from build123d import *

# Parameters (mm, degrees)
SKETCH1_R           = 2.25
BOSS_EXTRUDE1_DEPTH = 25
BOSS_EXTRUDE2_DEPTH = 4
CHAMFER1_SIZE       = 0.5


with BuildPart() as part:
    # Sketch1 → Boss-Extrude1 (new body)
    with BuildSketch(Plane.XY):
        Circle(SKETCH1_R)
    extrude(amount=BOSS_EXTRUDE1_DEPTH)

    # Sketch2 → Boss-Extrude2 (add)
    with BuildSketch(Plane.XY.offset(25)):
        Polygon((1.886184201, 3.57767771), (-2.155267683, 3.42232229), (-4.041451884, -0.15535542), (-1.886184201, -3.57767771), (2.155267683, -3.42232229), (4.041451884, 0.15535542), align=None)
    extrude(amount=BOSS_EXTRUDE2_DEPTH)

    # Sketch4 → Cut-Revolve1 (revolve, cut)
    with BuildSketch(Plane(origin=(0, 0, 0), x_dir=(1, 0, 0), z_dir=(0, 1, 0))):
        with BuildLine():
            Line((4.041451884, -28.3), (4.041451884, -29))
            Line((4.041451884, -29), (3.341451884, -29))
            ThreePointArc((3.341451884, -29), (3.836426631, -28.794974747), (4.041451884, -28.3))
        make_face()
    revolve(axis=Axis((-0.134541741, 0, 29), (0, 0, -1)), mode=Mode.SUBTRACT)

    # Chamfer1
    chamfer1_edges = [part.edges().sort_by_distance(p)[0] for p in [
        (-2.25, 0, 0),
    ]]
    chamfer(chamfer1_edges, length=CHAMFER1_SIZE)


solid = part.part
Build history of the part. All positions in model axes, mm. A direction names the side the tool comes from. Round coordinates to 2 decimals unless told otherwise and drop trailing zeros. Write each loop counter-clockwise with the first axis right and the second up, starting at its lowest first coordinate (ties: lowest second). Pieces come first, ordered by that corner, then holes. Notation, with made-up numbers: (60.25, 47.5) - (105.25, 47.5) arc R10 cw to (105.25, 53.5) - close; hole circle Ø7 at (42, 87.5). An arc over 180 degrees is marked (long way). Use CSV: the item, a comma, the result in double quotes.
(1) Wall check: line 1 (Z direction, x = 1.5, y = -2.5); line 2 (Z direction, x = 1.5, y = 1.5); line 3 (Y direction, x = 0.75, z = 12.5). Give the ranges that are in metal, low to high.
Response:
line 1,"25 to 29"
line 2,"0.37 to 29"
line 3,"-2.12 to 2.12"
(2) Band-saw the part on B-B (z = 7.25). Write the cut outline in (x, y).
Response:
outline,"circle Ø4.5 at (0, 0)"
(3) Pin check, flat tips, straight feed: P1, Ø3, axis at x = -1.5, z = 20.5, coming from the -Y side; P2, Ø1.5, axis at y = -1.5, z = 23.5, coming from the +X side; P3, Ø1.5, axis at x = 2, z = 17, coming from the +Y side. Stop position of each tip, or through.
Response:
P1,"y = -2.25"
P2,"x = 2.12"
P3,"y = 1.87"
(4) 3-axis set-ups, long thin cutter, end or side, ignore diameter. For faces 1 (the flat face through (2, -2, 25)), 2 (the flat face through (0, 0, 0)): which of +Z, -Z, +X, -X, +Y, -Y reach the whole face in a straight line?
Response:
face 1,"-Z"
face 2,"-Z, +X, -X, +Y, -Y"
(5) Band-saw the part on A-A (z = 26.25). Write the cut outline in (x, y), plus the area to 3 significant figures.
Response:
outline,"(-4.04, -0.16) - (-1.89, -3.58) - (2.16, -3.42) - (4.04, 0.16) - (1.89, 3.58) - (-2.16, 3.42) - close"
area,"42.5 mm²"
